Verification items for the finished model (mm, model axes). A direction names the side the tool comes from. Round coordinates to 2 decimals unless told otherwise and drop trailing zeros. Write each loop counter-clockwise with the first axis right and the second up, starting at its lowest first coordinate (ties: lowest second). Pieces come first, ordered by that corner, then holes. Notation, with made-up numbers: M 15,-21 L 66,-21 A30 ccw 66,10 Z; hole C 55,10.25 d3. An arc over 180 degrees is marked long. Answer in a Markdown table with one row per item. Add a question column.
1. Sectioned sample at A-A on x = 88.5. Record the cut outline in (y, z).
2. Go/stop test with flat-tipped pins: pin 1 Ø6 at (x, y) = (5, -1.5) entering from -Z; pin 2 Ø10 at (x, z) = (87.5, 63.5) entering from -Y; pin 3 Ø4 at (x, z) = (-44, -23) entering from +Y; pin 4 Ø2.5 at (x, z) = (-26, 47) entering from -Y. Record where each tip stops, or that it passes through.
3. Sectioned sample at B-B on z = 71. Record the cut outline in (x, y).
4. Sectioned sample at D-D on z = 7. Record the cut outline in (x, y).
5. Set-up check for faces 1 (the flat face through (1.68, -1.2, -81.76)), 2 (the flat face through (-2, 0, 4)): record each of +Z, -Z, +X, -X, +Y, -Y from which the full face is reachable in a straight line by a thin tool's end or side.
6. Material ranges on probe 1 along X at (y, z) = (0.9, 47); probe 2 along Z at (x, y) = (26, 2); probe 3 along Y at (x, z) = (60, 72), recorded low to high.
7. Sectioned sample at C-C on y = -3.25. Record the cut outline in (x, z), plus the area to 3 significant figures.
8. Draft check along X on faces 3 (the flat face through (-120, 1, -19)), 4 (the flat face through (120, 1, -19)), 5 (the flat face through (-2, 3, -1)), 6 (the flat face through (-116, 4, 58)). Enter one of: pulls with the +X half, pulls with the -X half, needs draft (parallel to the pull), parting line crosses it, or undercut.
```python
from build123d import *

# Parameters (mm, degrees)
SKETCH2_W             = 4.75
SKETCH2_H             = 65.25
BOSS_EXTRUDE3_DEPTH   = 4
BOSS_EXTRUDE3_2_DEPTH = 4
SKETCH2_W_2           = 100
SKETCH2_H_2           = 4.5
BOSS_EXTRUDE3_3_DEPTH = 4
BOSS_EXTRUDE3_4_DEPTH = 4
BOSS_EXTRUDE3_5_DEPTH = 4
SKETCH2_5_R           = 1.65
SKETCH2_5_W           = 4.75
SKETCH2_5_H           = 30
SKETCH2_5_W_2         = 30
SKETCH2_5_H_2         = 4.5
BOSS_EXTRUDE4_DEPTH   = 3
SKETCH3_W             = 240
SKETCH3_H             = 10
BOSS_EXTRUDE5_DEPTH   = 8
CUT_EXTRUDE1_DEPTH    = 241
FILLET2_R             = 3


with BuildPart() as part:
    # Sketch2 → Boss-Extrude3 (new body)
    with BuildSketch(Plane(origin=(0, 0, 0), x_dir=(1, 0, 0), z_dir=(0, 1, 0))):
        with Locations((-117.625, 49.875)):
            Rectangle(SKETCH2_W, SKETCH2_H)
    extrude(amount=BOSS_EXTRUDE3_DEPTH)



with BuildPart() as body_2:
    # Sketch2 → Boss-Extrude3 2 (new body)
    with BuildSketch(Plane(origin=(0, 0, 0), x_dir=(1, 0, 0), z_dir=(0, 1, 0))):
        Polygon((-80, -82.5), (-80, -78), (-115.25, -78), (-115.25, -12.75), (-120, -12.75), (-120, -82.5), align=None)
    extrude(amount=BOSS_EXTRUDE3_2_DEPTH)


with BuildPart() as body_3:
    # Sketch2 → Boss-Extrude3 3 (new body)
    with BuildSketch(Plane(origin=(0, 0, 0), x_dir=(1, 0, 0), z_dir=(0, 1, 0))):
        with Locations((0, -80.25)):
            Rectangle(SKETCH2_W_2, SKETCH2_H_2)
    extrude(amount=BOSS_EXTRUDE3_3_DEPTH)


with BuildPart() as body_4:
    # Sketch2 → Boss-Extrude3 4 (new body)
    with BuildSketch(Plane(origin=(0, 0, 0), x_dir=(1, 0, 0), z_dir=(0, 1, 0))):
        Polygon((115.25, -78), (80, -78), (80, -82.5), (120, -82.5), (120, -12.75), (115.25, -12.75), align=None)
    extrude(amount=BOSS_EXTRUDE3_4_DEPTH)


with BuildPart() as body_5:
    # Sketch2 → Boss-Extrude3 5 (new body)
    with BuildSketch(Plane(origin=(0, 0, 0), x_dir=(1, 0, 0), z_dir=(0, 1, 0))):
        with Locations((117.625, 49.875)):
            Rectangle(SKETCH2_W, SKETCH2_H)
    extrude(amount=BOSS_EXTRUDE3_5_DEPTH)


with BuildPart() as part_1:
    add(part.part)

    add(body_2.part)  # Boss-Extrude4 merges body 2

    add(body_3.part)  # Boss-Extrude4 merges body 3

    add(body_4.part)  # Boss-Extrude4 merges body 4

    add(body_5.part)  # Boss-Extrude4 merges body 5
    # Sketch2_5 → Boss-Extrude4 (add)
    with BuildSketch(Plane(origin=(0, 0, 0), x_dir=(1, 0, 0), z_dir=(0, 1, 0))):
        Polygon((50, -78), (80, -78), (115.25, -78), (115.25, -12.75), (115.25, 17.25), (115.25, 82.5), (-115.25, 82.5), (-115.25, 17.25), (-115.25, -12.75), (-115.25, -78), (-80, -78), (-50, -78), align=None)
        with Locations((-44, -47)):
            Circle(SKETCH2_5_R, mode=Mode.SUBTRACT)
        with Locations((-26, -47)):
            Circle(SKETCH2_5_R, mode=Mode.SUBTRACT)
        with Locations((-44, -23)):
            Circle(SKETCH2_5_R, mode=Mode.SUBTRACT)
        with Locations((-26, -23)):
            Circle(SKETCH2_5_R, mode=Mode.SUBTRACT)
        with Locations((26, -47)):
            Circle(SKETCH2_5_R, mode=Mode.SUBTRACT)
        with Locations((44, -47)):
            Circle(SKETCH2_5_R, mode=Mode.SUBTRACT)
        with Locations((26, -23)):
            Circle(SKETCH2_5_R, mode=Mode.SUBTRACT)
        with Locations((44, -23)):
            Circle(SKETCH2_5_R, mode=Mode.SUBTRACT)
        with Locations((-44, 23)):
            Circle(SKETCH2_5_R, mode=Mode.SUBTRACT)
        with Locations((-26, 23)):
            Circle(SKETCH2_5_R, mode=Mode.SUBTRACT)
        with Locations((-44, 47)):
            Circle(SKETCH2_5_R, mode=Mode.SUBTRACT)
        with Locations((-26, 47)):
            Circle(SKETCH2_5_R, mode=Mode.SUBTRACT)
        with Locations((26, 23)):
            Circle(SKETCH2_5_R, mode=Mode.SUBTRACT)
        with Locations((44, 23)):
            Circle(SKETCH2_5_R, mode=Mode.SUBTRACT)
        with Locations((26, 47)):
            Circle(SKETCH2_5_R, mode=Mode.SUBTRACT)
        with Locations((44, 47)):
            Circle(SKETCH2_5_R, mode=Mode.SUBTRACT)
        with Locations((-117.625, 2.25)):
            Rectangle(SKETCH2_5_W, SKETCH2_5_H)
        with Locations((-65, -80.25)):
            Rectangle(SKETCH2_5_W_2, SKETCH2_5_H_2)
        with Locations((65, -80.25)):
            Rectangle(SKETCH2_5_W_2, SKETCH2_5_H_2)
        with Locations((117.625, 2.25)):
            Rectangle(SKETCH2_5_W, SKETCH2_5_H)
    extrude(amount=BOSS_EXTRUDE4_DEPTH)

    # Sketch3 → Boss-Extrude5 (add)
    with BuildSketch(Plane.XZ):
        with Locations((0, -77.5)):
            Rectangle(SKETCH3_W, SKETCH3_H)
    extrude(amount=BOSS_EXTRUDE5_DEPTH)

    # Sketch4 → Cut-Extrude1 (cut, through all)
    with BuildSketch(Plane(origin=(120, 0, 0), x_dir=(0, 0, -1), z_dir=(1, 0, 0))):
        Polygon((82.5, 3), (80.560403212, -8), (82.5, -8), align=None)
    extrude(amount=-CUT_EXTRUDE1_DEPTH, mode=Mode.SUBTRACT)

    # Fillet2
    fillet2_edges = [part_1.edges().sort_by_distance(p)[0] for p in [
        (0, -8, -80.560403212),
    ]]
    fillet(fillet2_edges, radius=FILLET2_R)


solid = part_1.part
```
Geometry check:
| question | item | result |
|---|---|---|
| 1 | outline | M -8,-78.04 A3 ccw -5.52,-81 L 3,-82.5 L 3,78 L 4,78 L 4,82.5 L 0,82.5 L 0,-72.5 L -8,-72.5 Z |
| 2 | pin 1 | stops at z = -82.24 |
| 2 | pin 2 | stops at y = 0 |
| 2 | pin 3 | stops at y = 3 |
| 2 | pin 4 | passes through |
| 3 | outline | M -120,0 L 120,0 L 120,4 L 115.25,4 L 115.25,3 L -115.25,3 L -115.25,4 L -120,4 Z |
| 4 | outline | M -120,0 L 120,0 L 120,3 L -120,3 Z |
| 5 | face 1 | -Z, +X, -X, -Y |
| 5 | face 2 | +Z, +X, -X, -Y |
| 6 | probe 1 | x = -120 to -45.65, -42.35 to -27.65, -24.35 to 24.35, 27.65 to 42.35, 45.65 to 120 |
| 6 | probe 2 | z = -82.32 to -48.65, -45.35 to -24.65, -21.35 to 21.35, 24.65 to 45.35, 48.65 to 82.5 |
| 6 | probe 3 | y = 0 to 3 |
| 7 | outline | M -120,-81.4 L 120,-81.4 L 120,-72.5 L -120,-72.5 Z |
| 7 | area | 2,140 mm2 |
| 8 | face 3 | pulls with the -X half |
| 8 | face 4 | pulls with the +X half |
| 8 | face 5 | undercut |
| 8 | face 6 | needs draft |
